```python
from build123d import *

# Parameters (mm, degrees)
SKETCH1_R           = 2.286
SKETCH1_R_2         = 1.905
SKETCH1_R_3         = 4.7625
BOSS_EXTRUDE1_DEPTH = 6.35
SKETCH2_R           = 1.905
CUT_EXTRUDE1_DEPTH  = 7.9375


with BuildPart() as part:
    # Sketch1 → Boss-Extrude1 (new body)
    with BuildSketch(Plane.XY):
        with BuildLine():
            Line((35.017380191, 51.909842308), (36.511130592, 114.185799576))
            ThreePointArc((36.511130592, 114.185799576), (34.05178904, 118.469313309), (29.116569093, 118.26817942))
            Line((29.116569093, 118.26817942), (3.81, 101.473802417))
            Line((3.81, 101.473802417), (3.81, 46.529605935))
            Line((3.81, 46.529605935), (-6.095047303, 1.78126314))
            ThreePointArc((-6.095047303, 1.78126314), (-2.403049878, -5.877742023), (5.597196577, -2.998981573))
            Line((5.597196577, -2.998981573), (35.017380191, 51.909842308))
        make_face()
        Circle(SKETCH1_R, mode=Mode.SUBTRACT)
        with Locations((31.75, 114.3)):
            Circle(SKETCH1_R_2, mode=Mode.SUBTRACT)
        with Locations((22.225, 59.483605935)):
            Circle(SKETCH1_R_3, mode=Mode.SUBTRACT)
    extrude(amount=BOSS_EXTRUDE1_DEPTH)

    # Sketch2 → Cut-Extrude1 (cut)
    with BuildSketch(Plane.ZY.offset(-3.81)):
        with Locations(Location((3.175, 89.876704176, 0), (0, 0, 270))):
            Circle(SKETCH2_R)
        with Locations(Location((3.175, 58.126704176, 0), (0, 0, 270))):
            Circle(SKETCH2_R)
    extrude(amount=-CUT_EXTRUDE1_DEPTH, mode=Mode.SUBTRACT)


solid = part.part
```
Build history of the part. All positions in model axes, mm. A direction names the side the tool comes from. Give positions to 0.01 mm unless a question says otherwise; leave off trailing zeros. Order: outer loops, then holes, each group sorted by start corner. A loop starts at its lowest first (then second) coordinate and runs counter-clockwise, first axis right, second up. Notation, with made-up numbers: M 39,-22.75 L 68,-22.75 A15 cw 68,-4.75 Z; hole C 60,84.5 d11. An arc over 180 degrees is marked long. Write item = value, one per line. Start each with the question number.
(1) Slice it at C-C on x = 9. Write the cut outline in (y, z) (3 decimals).
(2) Probe L1, parallel to Y at x = 10, z = 2.5; L2, parallel to Y at x = 31.75, z = 1.75 (1 decimal); L3, parallel to Y at x = 5.5, z = 3.5. List the from-to ranges inside material, lowest first. Write a range as [from, to].
(3) Slice it at A-A on x = 0. Write the cut outline in (y, z).
(4) Pin check, flat tips, straight feed: pin 1 Ø3 at (y, z) = (89.5, 3.5) entering from -X; pin 2 Ø3 at (x, z) = (20, 2.5) entering from +Y; pin 3 Ø3 at (y, z) = (89.88, 3.18) entering from -X. Stop position of each tip, or through.
(5) Slice it at B-B on y = 0. Write the cut outline in (x, z), plus the area to 3 significant figures.
(6) Slice it at D-D on y = 104.5. Write the cut outline in (x, z), plus the area to 3 significant figures.
(7) Two-plate mould, pull along Y, no slides. Class faces 4 (the flat face through (11.748, 90, 3)), 5 (the flat face through (15, 57, 0)), 6 (the flat face through (16.64, 109.99, 3.13)): released by +Y, released by -Y, zero draft, split by the parting line, or undercut.
(8) Which spindle directions (+Z, -Z, +X, -X, +Y, -Y) get a long thin tool onto all of the face, cutting with end or side? Do faces 1 (the cylindrical face through (31.5, 116.19, 3.13)), 2 (the flat face through (3.81, 74, 3)), 3 (the cylindrical face through (7.72, 91.78, 3.26)). Say none if no direction does.
Responses:
q1.outline = M 3.352,0 L 104.918,0 L 104.918,6.35 L 3.352,6.35 Z; hole C 58.127,3.175 d3.81; hole C 89.877,3.175 d3.81
q2.L1 = [5.22, 56.35], [59.91, 88.1], [91.66, 105.58]
q2.L2 = [45.8, 112.4], [116.2, 119.1]
q2.L3 = [-3.17, 56.25], [60, 88], [91.75, 102.6]
q3.outline = M -6.35,0 L -2.29,0 L -2.29,6.35 L -6.35,6.35 Z; M 2.29,0 L 29.32,0 L 29.32,6.35 L 2.29,6.35 Z
q4.pin_1 = 3.81
q4.pin_2 = 113.21
q4.pin_3 = 11.75
q5.outline = M -6.35,0 L -2.29,0 L -2.29,6.35 L -6.35,6.35 Z; M 2.29,0 L 7.2,0 L 7.2,6.35 L 2.29,6.35 Z
q5.area = 57.0 mm2
q6.outline = M 8.37,0 L 36.28,0 L 36.28,6.35 L 8.37,6.35 Z
q6.area = 177 mm2
q7.face_4 = undercut
q7.face_5 = zero draft
q7.face_6 = released by +Y
q8.face_1 = +Z, -Z
q8.face_2 = +Z, -Z, -X, +Y
q8.face_3 = -X
